Source: three-view drawing plus pictorial views. Frame: mm from the lowest corner of the part. Round coordinates to 2 decimals unless told otherwise and drop trailing zeros. Loops run counter-clockwise (first coordinate to the right, second up) from the corner with the lowest first, then second, coordinate; pieces in that order, holes last. Notation, with made-up numbers: (41, 58.5) -> (67, 58.5) arc R5 cw to (67, 63.5) -> close; hole circle Ø5 at (12.5, -40). An arc over 180 degrees is marked (long way). Put each result on its own line as item: value. Start each with the question number.
1. Cut plane C-C (y = 71). Return the cut outline in (x, z).
2. Draft query along X for the marked faces 1, 2 and 3. Return one class per face: pulls with the +X half, pulls with the -X half, needs draft (parallel to the pull), parting line crosses it, or undercut.
3. Cut plane D-D (x = 14). Return the cut outline in (y, z).
4. Cut plane A-A (y = 13.85). Return the cut outline in (x, z).
5. Material intervals for L1, parallel to Z at x = 1.65, y = 13.85; L2, parallel to Y at x = 9, z = 1.9; L3, parallel to X at y = 39, z = 14, sorted ascending.
6. Cut plane B-B (z = 25). Return the cut outline in (x, y), then the cut area to 3 significant figures.
7. Contact query for flat-ended pins moving along their axis: pin 1 (6 mm diameter, centred on y = 52.5, z = 23.5, fed in from +X); pin 2 (2.5 mm diameter, centred on y = 75.85, z = 25, fed in from -X); pin 3 (4 mm diameter, centred on x = 10.3, y = 79.7, fed in from +Z). Output: stop coordinate, or through.
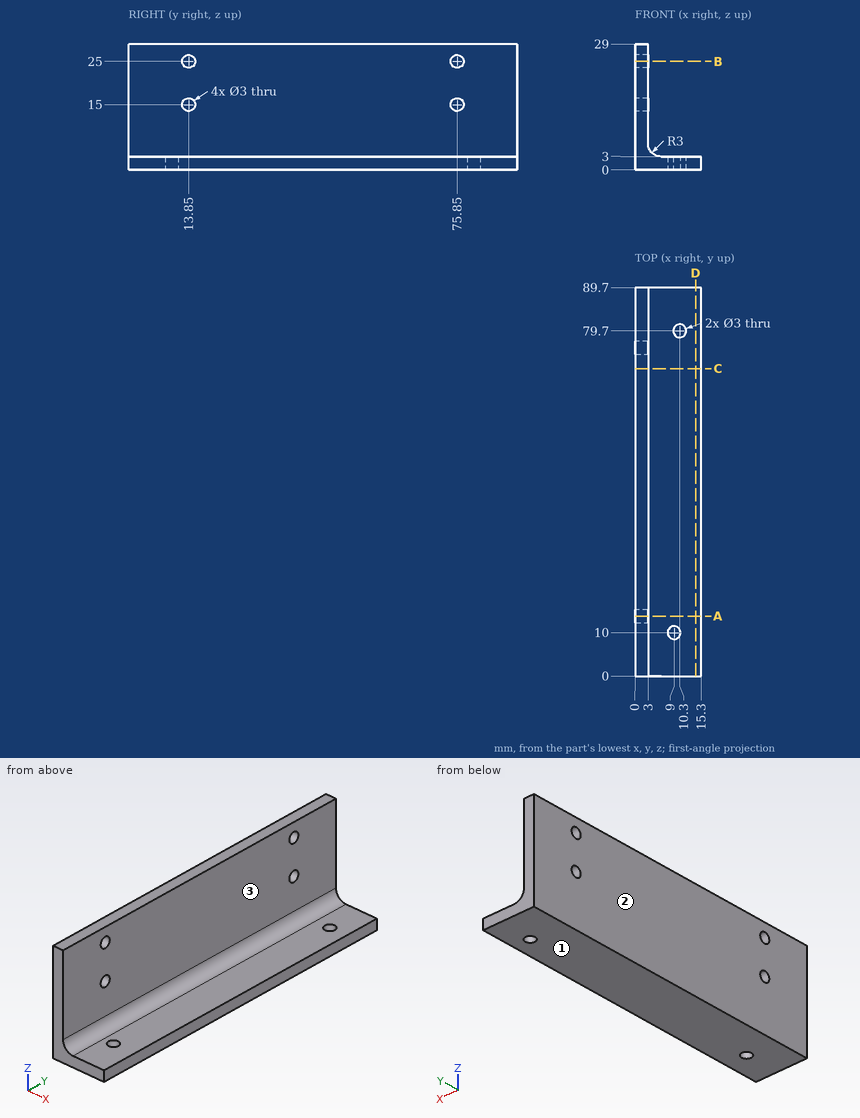
Solution:
1. outline: (0, 0) -> (15.3, 0) -> (15.3, 3) -> (6, 3) arc R3 cw to (3, 6) -> (3, 29) -> (0, 29) -> close
2. face 1: needs draft
2. face 2: pulls with the -X half
2. face 3: pulls with the +X half
3. outline: (0, 0) -> (89.7, 0) -> (89.7, 3) -> (0, 3) -> close
4. outline: (0, 0) -> (15.3, 0) -> (15.3, 3) -> (6, 3) arc R3 cw to (3, 6) -> (3, 13.5) -> (0, 13.5) -> close; (0, 16.5) -> (3, 16.5) -> (3, 23.5) -> (0, 23.5) -> close; (0, 26.5) -> (3, 26.5) -> (3, 29) -> (0, 29) -> close
5. L1: z = 0 to 13.5, 16.5 to 23.5, 26.5 to 29
5. L2: y = 0 to 8.5, 11.5 to 78.95, 80.45 to 89.7
5. L3: x = 0 to 3
6. outline: (0, 0) -> (3, 0) -> (3, 12.35) -> (0, 12.35) -> close; (0, 15.35) -> (3, 15.35) -> (3, 74.35) -> (0, 74.35) -> close; (0, 77.35) -> (3, 77.35) -> (3, 89.7) -> (0, 89.7) -> close
6. area: 251 mm^2
7. pin 1: stops at x = 3
7. pin 2: passes through
7. pin 3: stops at z = 3
